The figure shows three views and two pictorial views of one solid part (mm, origin at its lowest corner). Answer the questions. A direction names the side the tool comes from. Round coordinates to 2 decimals unless told otherwise and drop trailing zeros. Order: outer loops, then holes, each group sorted by start corner. A loop starts at its lowest first (then second) coordinate and runs counter-clockwise, first axis right, second up. Notation, with made-up numbers: (8, 57) -> (33, 57) arc R32 ccw to (33, 85) -> close; hole circle Ø2 at (61, -27). An arc over 180 degrees is marked (long way). Return JSON: item names as keys, results as strings. Group by question number.
(1) The part is cut by section C-C (y = 11.5). Determine the outline of the cut face in (x, z), plus the area to 3 significant figures.
(2) Consider line 1 (Y direction, x = 17, z = 2.2); line 2 (Z direction, x = 5.5, y = 10); line 3 (Y direction, x = 17, z = 1.2). Determine where each line is inside the solid, lowest interval first. Write a range as [from, to].
(3) Each of these flat-tipped pins is pushed along its axis until it touches: pin 1 (1.5 mm diameter, centred on x = 6, z = 4, fed in from +Y); pin 2 (1 mm diameter, centred on y = 24.5, z = 5.5, fed in from -X); pin 3 (4 mm diameter, centred on y = 6.5, z = 2, fed in from -X); pin 4 (3 mm diameter, centred on x = 17, y = 17, fed in from +Z). Where does it stop, or does it pass through?
(4) Which of the six approach directions +Z, -Z, +X, -X, +Y, -Y give full straight-line access (tool end or side, diameter ignored) to the marked faces 1 and 2?
(5) The part is cut by section A-A (y = 17). Determine the outline of the cut face in (x, z), plus the area to 3 significant figures.
(6) Determine the mould class of the marked faces 3, 4 and 5 for opening direction Y: +Y half, -Y half, draft (parallel to the pull), parting line (faces both ways), or undercut.
(7) The part is cut by section D-D (x = 10). Determine the outline of the cut face in (y, z).
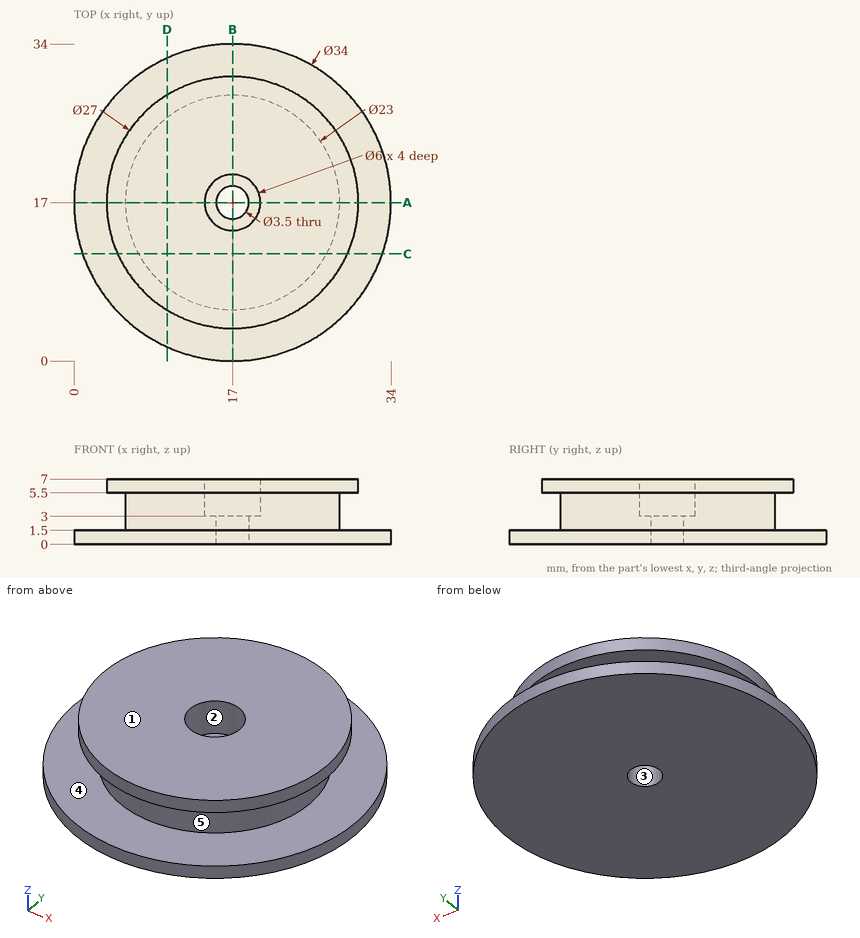
Answer below:
{
 "1": {"outline": "(0.91, 0) -> (33.09, 0) -> (33.09, 1.5) -> (27.1, 1.5) -> (27.1, 5.5) -> (29.33, 5.5) -> (29.33, 7) -> (4.67, 7) -> (4.67, 5.5) -> (6.9, 5.5) -> (6.9, 1.5) -> (0.91, 1.5) -> close", "area": "166 mm²"},
 "2": {"line 1": "y = [5.5, 15.25], [18.75, 28.5]", "line 2": "z = [0, 1.5], [5.5, 7]", "line 3": "y = [0, 15.25], [18.75, 34]"},
 "3": {"pin 1": "stops at y = 22.21", "pin 2": "stops at x = 5.46", "pin 3": "stops at x = 2.31", "pin 4": "passes through"},
 "4": {"face 1": "+Z, +X, -X, +Y, -Y", "face 2": "+Z"},
 "5": {"outline": "(0, 0) -> (15.25, 0) -> (15.25, 3) -> (14, 3) -> (14, 7) -> (3.5, 7) -> (3.5, 5.5) -> (5.5, 5.5) -> (5.5, 1.5) -> (0, 1.5) -> close; (18.75, 0) -> (34, 0) -> (34, 1.5) -> (28.5, 1.5) -> (28.5, 5.5) -> (30.5, 5.5) -> (30.5, 7) -> (20, 7) -> (20, 3) -> (18.75, 3) -> close", "area": "149 mm²"},
 "6": {"face 3": "undercut", "face 4": "draft", "face 5": "parting line"},
 "7": {"outline": "(1.51, 0) -> (32.49, 0) -> (32.49, 1.5) -> (26.12, 1.5) -> (26.12, 5.5) -> (28.54, 5.5) -> (28.54, 7) -> (5.46, 7) -> (5.46, 5.5) -> (7.88, 5.5) -> (7.88, 1.5) -> (1.51, 1.5) -> close"}
}
